Check sheet for the drawn part. Datum: minimum x, y, z corner. Units: mm. A direction names the side the tool comes from. Give positions to 0.01 mm unless a question says otherwise; leave off trailing zeros. Loops run counter-clockwise (first coordinate to the right, second up) from the corner with the lowest first, then second, coordinate; pieces in that order, holes last.
1. Material ranges on L1, parallel to X at y = 5.5, z = 30 (3 decimals); L2, parallel to Z at x = 1, y = 12.5; L3, parallel to Y at x = 2.5, z = 65, recorded low to high.
2. Tool access check on the marked faces 1 and 2. Record the directions out of +Z, -Z, +X, -X, +Y, -Y that give a thin tool (end or side, any length) a straight path to the whole face; none if there is none.
3. Cross-section at C-C, the plane x = 15.25. Record the cut outline in (y, z).
4. Cross-section at A-A, the plane y = 7.5. Record the cut outline in (x, z) (3 decimals).
5. Go/stop test with flat-tipped pins: pin 1 Ø5 at (x, z) = (11.5, 74) entering from -Y; pin 2 Ø3 at (x, y) = (17.5, 11.5) entering from -Z. Record where each tip stops, or that it passes through.
6. Release check for a two-part mould opening along X. For the marked faces 3, 4 and 5 record: +X half, -X half, draft (parallel to the pull), parting line (faces both ways), or undercut.
7. Cross-section at B-B, the plane z = 48. Record the cut outline in (x, y) (3 decimals), plus the area to 3 significant figures.
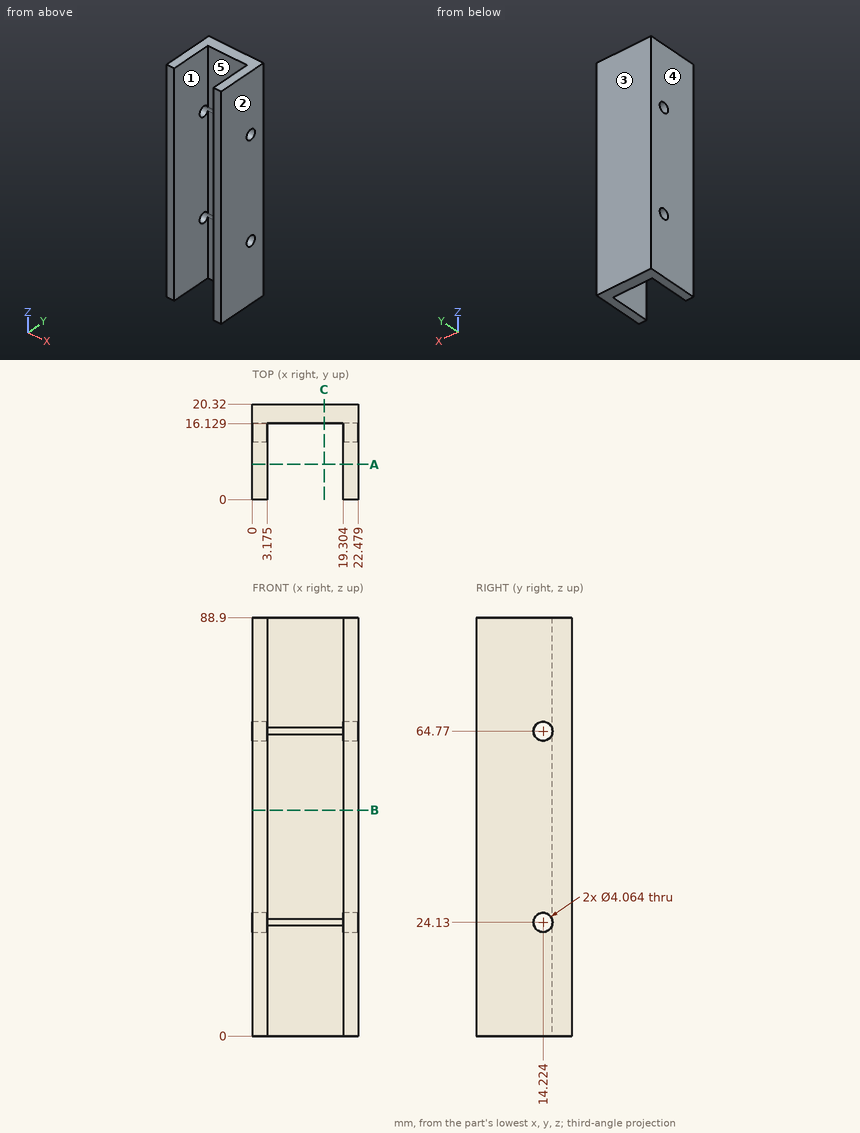
Result:
1. L1: x = 0 to 3.175, 19.304 to 22.479
1. L2: z = 0 to 23.05, 25.21 to 63.69, 65.85 to 88.9
1. L3: y = 0 to 12.21, 16.24 to 20.32
2. face 1: +Z, -Z, -Y
2. face 2: +Z, -Z, +X, +Y, -Y
3. outline: (16.13, 0) - (20.32, 0) - (20.32, 88.9) - (16.13, 88.9) - (16.13, 65.48) arc R2.03 cw to (16.13, 64.06) - (16.13, 24.84) arc R2.03 cw to (16.13, 23.42) - close
4. outline: (0, 0) - (3.175, 0) - (3.175, 88.9) - (0, 88.9) - close; (19.304, 0) - (22.479, 0) - (22.479, 88.9) - (19.304, 88.9) - close
5. pin 1: stops at y = 16.13
5. pin 2: passes through
6. face 3: draft
6. face 4: -X half
6. face 5: undercut
7. outline: (0, 0) - (3.175, 0) - (3.175, 16.129) - (19.304, 16.129) - (19.304, 0) - (22.479, 0) - (22.479, 20.32) - (0, 20.32) - close
7. area: 197 mm2
